```python
from build123d import *

# Parameters (mm, degrees)
SKETCH1_W           = 85
SKETCH1_H           = 80
BOSS_EXTRUDE1_DEPTH = 5
SKETCH2_R           = 1.5
CUT_EXTRUDE1_DEPTH  = 59.576872569
BOSS_EXTRUDE3_DEPTH = 30
SKETCH5_R           = 3.5
CUT_EXTRUDE2_DEPTH  = 2
SKETCH6_R           = 1.25
CUT_EXTRUDE3_DEPTH  = 101.249688279
SKETCH3_W           = 85
SKETCH3_H           = 80
BOSS_EXTRUDE4_DEPTH = 10


with BuildPart() as part:
    # Sketch1 → Boss-Extrude1 (new body)
    with BuildSketch(Plane(origin=(0, 0, 0), x_dir=(1, 0, 0), z_dir=(0, 1, 0))):
        Rectangle(SKETCH1_W, SKETCH1_H)
    extrude(amount=BOSS_EXTRUDE1_DEPTH)

    # Sketch2 → Cut-Extrude1 (cut, through all)
    with BuildSketch(Plane.XZ):
        with Locations(Location((0, 19.6, 0), (0, 0, 270))):
            Circle(SKETCH2_R)
        with Locations(Location((0, -19.6, 0), (0, 0, 90))):
            Circle(SKETCH2_R)
    extrude(amount=-CUT_EXTRUDE1_DEPTH, mode=Mode.SUBTRACT)

    # Sketch4 → Boss-Extrude3 (add)
    with BuildSketch(Plane(origin=(0, 5, 0), x_dir=(1, 0, 0), z_dir=(0, 1, 0))):
        Polygon((-42.5, -40), (-42.5, 40), (-37.5, 40), (-37.5, -35), (37.5, -35), (37.5, 40), (42.5, 40), (42.5, -40), align=None)
    extrude(amount=BOSS_EXTRUDE3_DEPTH)

    # Sketch5 → Cut-Extrude2 (cut)
    with BuildSketch(Plane(origin=(0, 5, 0), x_dir=(1, 0, 0), z_dir=(0, 1, 0))):
        with Locations(Location((0, 19.6, 0), (0, 0, 270))):
            Circle(SKETCH5_R)
        with Locations(Location((0, -19.6, 0), (0, 0, 270))):
            Circle(SKETCH5_R)
    extrude(amount=-CUT_EXTRUDE2_DEPTH, mode=Mode.SUBTRACT)

    # Sketch6 → Cut-Extrude3 (cut, through all)
    with BuildSketch(Plane.ZY.offset(42.5)):
        with Locations((10.624581332, 2.504153155)):
            Circle(SKETCH6_R)
        with Locations((3.123107186, 18.591116375)):
            Circle(SKETCH6_R)
        Polygon((24.335207615, 35), (-40, 5), (-40, 35), align=None)
    extrude(amount=-CUT_EXTRUDE3_DEPTH, mode=Mode.SUBTRACT)

    # Sketch3 → Boss-Extrude4 (add)
    with BuildSketch(Plane.XZ):
        Rectangle(SKETCH3_W, SKETCH3_H)
        Polygon((29.5, -17), (32, -17), (32, -5), (29.5, -5), (29.5, 24), (-29.5, 24), (-29.5, -24), (29.5, -24), align=None, mode=Mode.SUBTRACT)
    extrude(amount=BOSS_EXTRUDE4_DEPTH)


solid = part.part
```
Geometry check sheet. Reference: the model listing, model coordinates, mm. A direction names the side the tool comes from. Coordinates: 2 decimals unless noted, no trailing zeros. Order: outer loops, then holes, each group sorted by start corner. A loop starts at its lowest first (then second) coordinate and runs counter-clockwise, first axis right, second up.
Q1. Thickness scan on probe 1 along X at (y, z) = (-0.5, -9.5); probe 2 along X at (y, z) = (22, 20); probe 3 along Y at (x, z) = (23.5, -4.5). Record the ranges inside material, lowest first.
Reply:
probe 1: x = -42.5 to -29.5, 32 to 42.5
probe 2: x = -42.5 to -37.5, 37.5 to 42.5
probe 3: y = 0 to 5
Q2. Depth check by flat-ended pin: pin 1 Ø2 at (x, y) = (3.5, 18.5) entering from -Z; pin 2 Ø7.5 at (x, z) = (1.5, 18) entering from +Y; pin 3 Ø2 at (x, z) = (1.5, -19.5) entering from +Y. Enter the tip coordinate at first touch or a pass-through.
Reply:
pin 1: stops at z = 35
pin 2: stops at y = 5
pin 3: stops at y = 3
Q3. Sectioned sample at A-A on x = 0. Record the cut outline in (y, z), and give its area (3 significant figures).
Reply:
outline: (-10, -40) - (5, -40) - (5, -23.1) - (3, -23.1) - (3, -21.1) - (0, -21.1) - (0, -24) - (-10, -24) - close; (-10, 24) - (0, 24) - (0, 21.1) - (3, 21.1) - (3, 23.1) - (5, 23.1) - (5, 35) - (35, 35) - (35, 40) - (-10, 40) - close; (0, -18.1) - (3, -18.1) - (3, -16.1) - (5, -16.1) - (5, 16.1) - (3, 16.1) - (3, 18.1) - (0, 18.1) - close; hole circle Ø2.5 at (2.5, 10.62)
area: 819 mm2
Q4. Sectioned sample at C-C on y = -5. Record the cut outline in (x, z).
Reply:
outline: (-42.5, -40) - (42.5, -40) - (42.5, 40) - (-42.5, 40) - close; hole (-29.5, -24) - (29.5, -24) - (29.5, -17) - (32, -17) - (32, -5) - (29.5, -5) - (29.5, 24) - (-29.5, 24) - close
Q5. Sectioned sample at D-D on x = -27. Record the cut outline in (y, z), and give its area (3 significant figures).
Reply:
outline: (-10, -40) - (5, -40) - (5, 35) - (35, 35) - (35, 40) - (-10, 40) - (-10, 24) - (0, 24) - (0, -24) - (-10, -24) - close; hole circle Ø2.5 at (2.5, 10.62)
area: 865 mm2
Q6. Tool access check on faces 4 (the face through (29.5, -5, -21)), 5 (the face through (-37.5, 16, 5)), 6 (the face through (0.154, 4.014, 16.103)), 7 (the face through (40, 20.2, -7.4)). Record the directions out of +Z, -Z, +X, -X, +Y, -Y that give a thin tool (end or side, any length) a straight path to the whole face; none if there is none.
Reply:
face 4: -Y
face 5: -Z, +Y
face 6: +Y
face 7: -Z, +X, -X, +Y
Q7. Sectioned sample at B-B on z = 19.6. Record the cut outline in (x, y).
Reply:
outline: (-42.5, -10) - (-29.5, -10) - (-29.5, 0) - (-1.5, 0) - (-1.5, 3) - (-3.5, 3) - (-3.5, 5) - (-37.5, 5) - (-37.5, 32.79) - (-42.5, 32.79) - close; (1.5, 0) - (29.5, 0) - (29.5, -10) - (42.5, -10) - (42.5, 32.79) - (37.5, 32.79) - (37.5, 5) - (3.5, 5) - (3.5, 3) - (1.5, 3) - close
Q8. Draft check along Y on faces 1 (the face through (39.97, 17.37, 2.85)), 2 (the face through (-40, 20.2, -7.4)), 3 (the face through (-42.5, 8, 8)). Enter one of: released by +Y, released by -Y, zero draft, split by the parting line, or undercut.
Reply:
face 1: undercut
face 2: released by +Y
face 3: zero draft
